Design review of the part built by this model. Coordinates are the model's own, in mm. Give positions to 0.01 mm unless a question says otherwise; leave off trailing zeros. Order: outer loops, then holes, each group sorted by start corner. A loop starts at its lowest first (then second) coordinate and runs counter-clockwise, first axis right, second up. Notation, with made-up numbers: (-3.75, 8) - (21.25, 8) arc R18 ccw to (21.25, 33) - close; hole circle Ø2 at (20.25, 53.25). An arc over 180 degrees is marked (long way). Write each question's results on one line, items separated by ' | '. Start each with the question number.
```python
from build123d import *

# Parameters (mm, degrees)
SKETCH1_W               = 510
SKETCH1_H               = 350
BOSS_EXTRUDE1_DEPTH     = 5
SKETCH2_R               = 5
SKETCH2_R_2             = 2.5
F_1_JOYYSTICK_DEPTH     = 619.566892098
SKETCH3_R               = 12
F_1_BUTTONS_DEPTH       = 619.566892098
SKETCH4_R               = 6.25
F_1_ROCKET_SWITCH_DEPTH = 619.566892098
SKETCH5_R               = 2.25
SKETCH5_W               = 2
SKETCH5_H               = 74
F_1_POTENTIOMETER_DEPTH = 619.566892098
FILLET1_R               = 35
SKETCH6_R               = 12
F_2_BUTTONS_DEPTH       = 619.566892098
SKETCH9_R               = 25
F_2_SPEAKER_DEPTH       = 619.566892098
SKETCH10_R              = 6.25
F_2_ROCKET_SWITCH_DEPTH = 619.566892098
SKETCH8_R               = 2
SKETCH8_W               = 2
SKETCH8_H               = 75
F_2_POTENTIOMETER_DEPTH = 619.566892098


with BuildPart() as part:
    # Sketch1 → Boss-Extrude1 (new body)
    with BuildSketch(Plane(origin=(0, 0, 0), x_dir=(1, 0, 0), z_dir=(0, 1, 0))):
        with Locations((255, 175)):
            Rectangle(SKETCH1_W, SKETCH1_H)
    extrude(amount=BOSS_EXTRUDE1_DEPTH)

    # Sketch2 → 1 Joyystick (cut, through all)
    with BuildSketch(Plane(origin=(0, 5, 0), x_dir=(1, 0, 0), z_dir=(0, 1, 0))):
        with Locations(Location((120, 250, 0), (0, 0, 270))):
            Circle(SKETCH2_R)
        with Locations(Location((162.5, 270, 0), (0, 0, 270))):
            Circle(SKETCH2_R_2)
        with Locations(Location((162.5, 230, 0), (0, 0, 90))):
            Circle(SKETCH2_R_2)
        with Locations(Location((77.5, 230, 0), (0, 0, 270))):
            Circle(SKETCH2_R_2)
        with Locations(Location((77.5, 270, 0), (0, 0, 90))):
            Circle(SKETCH2_R_2)
    extrude(amount=-F_1_JOYYSTICK_DEPTH, mode=Mode.SUBTRACT)

    # Sketch3 → 1 Buttons (cut, through all)
    with BuildSketch(Plane(origin=(0, 5, 0), x_dir=(1, 0, 0), z_dir=(0, 1, 0))):
        with Locations(Location((80, 180, 0), (0, 0, 270))):
            Circle(SKETCH3_R)
        with Locations(Location((130, 180, 0), (0, 0, 270))):
            Circle(SKETCH3_R)
        with Locations(Location((100, 130, 0), (0, 0, 270))):
            Circle(SKETCH3_R)
        with Locations(Location((150, 130, 0), (0, 0, 270))):
            Circle(SKETCH3_R)
        with Locations(Location((150, 80, 0), (0, 0, 270))):
            Circle(SKETCH3_R)
    extrude(amount=-F_1_BUTTONS_DEPTH, mode=Mode.SUBTRACT)

    # Sketch4 → 1 Rocket Switch (cut, through all)
    with BuildSketch(Plane(origin=(0, 5, 0), x_dir=(1, 0, 0), z_dir=(0, 1, 0))):
        with Locations(Location((190, 280, 0), (0, 0, 270))):
            Circle(SKETCH4_R)
    extrude(amount=-F_1_ROCKET_SWITCH_DEPTH, mode=Mode.SUBTRACT)

    # Sketch5 → 1 Potentiometer (cut, through all)
    with BuildSketch(Plane(origin=(0, 5, 0), x_dir=(1, 0, 0), z_dir=(0, 1, 0))):
        with Locations(Location((178.719749064, 192, 0), (0, 0, 270))):
            Circle(SKETCH5_R)
        with Locations(Location((192.718338039, 191.801237073, 0), (0, 0, 90))):
            Circle(SKETCH5_R)
        with Locations(Location((192.718338039, 108.198762927, 0), (0, 0, 270))):
            Circle(SKETCH5_R)
        with Locations(Location((178.719749064, 108, 0), (0, 0, 90))):
            Circle(SKETCH5_R)
        with Locations((191, 150)):
            Rectangle(SKETCH5_W, SKETCH5_H)
    extrude(amount=-F_1_POTENTIOMETER_DEPTH, mode=Mode.SUBTRACT)

    # Fillet1
    fillet1_edges = [part.edges().sort_by_distance(p)[0] for p in [
        (0, 2.5, -350),
        (510, 2.5, -350),
        (510, 2.5, 0),
        (0, 2.5, 0),
    ]]
    fillet(fillet1_edges, radius=FILLET1_R)

    # Sketch6 → 2 Buttons (cut, through all)
    with BuildSketch(Plane(origin=(0, 5, 0), x_dir=(1, 0, 0), z_dir=(0, 1, 0))):
        with Locations(Location((460, 200, 0), (0, 0, 270))):
            Circle(SKETCH6_R)
        with Locations(Location((410, 200, 0), (0, 0, 270))):
            Circle(SKETCH6_R)
        with Locations(Location((424.025675508, 150, 0), (0, 0, 270))):
            Circle(SKETCH6_R)
        with Locations(Location((374.025675508, 150, 0), (0, 0, 270))):
            Circle(SKETCH6_R)
        with Locations(Location((460, 110, 0), (0, 0, 270))):
            Circle(SKETCH6_R)
    extrude(amount=-F_2_BUTTONS_DEPTH, mode=Mode.SUBTRACT)

    # Sketch9 → 2 speaker (cut, through all)
    with BuildSketch(Plane(origin=(0, 5, 0), x_dir=(1, 0, 0), z_dir=(0, 1, 0))):
        with Locations(Location((410, 290, 0), (0, 0, 270))):
            Circle(SKETCH9_R)
    extrude(amount=-F_2_SPEAKER_DEPTH, mode=Mode.SUBTRACT)

    # Sketch10 → 2 Rocket Switch (cut, through all)
    with BuildSketch(Plane(origin=(0, 5, 0), x_dir=(1, 0, 0), z_dir=(0, 1, 0))):
        with Locations(Location((370, 80, 0), (0, 0, 270))):
            Circle(SKETCH10_R)
    extrude(amount=-F_2_ROCKET_SWITCH_DEPTH, mode=Mode.SUBTRACT)

    # Sketch8 → 2 Potentiometer (cut, through all)
    with BuildSketch(Plane(origin=(0, 5, 0), x_dir=(1, 0, 0), z_dir=(0, 1, 0))):
        with Locations(Location((320, 192.5, 0), (0, 0, 270))):
            Circle(SKETCH8_R)
        with Locations(Location((320, 107.5, 0), (0, 0, 90))):
            Circle(SKETCH8_R)
        with Locations(Location((306, 107.5, 0), (0, 0, 270))):
            Circle(SKETCH8_R)
        with Locations(Location((306, 192.5, 0), (0, 0, 90))):
            Circle(SKETCH8_R)
        with Locations((308, 150)):
            Rectangle(SKETCH8_W, SKETCH8_H)
    extrude(amount=-F_2_POTENTIOMETER_DEPTH, mode=Mode.SUBTRACT)


solid = part.part
```
Q1. For line 1 (X direction, y = 2.1, z = -151); line 2 (Z direction, x = 162.5, y = 3.8); line 3 (X direction, y = 2.5, z = -230), list the stretches that pass through material, from the lowest coordinate up. Write a range as [from, to].
Q2. Add section A-A (x = 150). Give the boundary of the cut face in (y, z).
Q3. Add section B-B (z = -130). Give the boundary of the cut face in (x, y).
Q4. Add section C-C (z = -200). Give the boundary of the cut face in (x, y), plus the area to 3 significant figures.
Q5. Draft analysis for pull direction Z (two halves, no side actions). For faces 1 (the cylindrical face through (499.475, 2.535, -9.981)), 2 (the flat face through (251, 0, -177)), 3 (the cylindrical face through (468.11, 2.535, -118.844)), 4 (the cylindrical face through (499.475, 2.535, -340.019)), state which applies: pulls with the +Z half, pulls with the -Z half, needs draft (parallel to the pull), parting line crosses it, or undercut.
Q6. Insertion check: pin 1 Ø2.5 at (x, z) = (178.72, -108) entering from -Y. The pin has a flat end and moves straight along its axis. Give the tip position at first contact, or say it passes through.
Q7. Add section D-D (z = -296). Give the boundary of the cut face in (x, y).
Verdict:
1) line 1: x = [0, 190], [192, 307], [309, 362.07], [385.98, 412.07], [435.98, 510] | line 2: z = [-350, -272.5], [-267.5, -232.5], [-227.5, 0] | line 3: x = [0, 75], [80, 160], [165, 510]
2) outline: (0, -350) - (5, -350) - (5, -142) - (0, -142) - close; (0, -118) - (5, -118) - (5, -92) - (0, -92) - close; (0, -68) - (5, -68) - (5, 0) - (0, 0) - close
3) outline: (0, 0) - (88, 0) - (88, 5) - (0, 5) - close; (112, 0) - (138, 0) - (138, 5) - (112, 5) - close; (162, 0) - (190, 0) - (190, 5) - (162, 5) - close; (192, 0) - (307, 0) - (307, 5) - (192, 5) - close; (309, 0) - (510, 0) - (510, 5) - (309, 5) - close
4) outline: (0, 0) - (398, 0) - (398, 5) - (0, 5) - close; (422, 0) - (448, 0) - (448, 5) - (422, 5) - close; (472, 0) - (510, 0) - (510, 5) - (472, 5) - close | area: 2,310 mm2
5) face 1: pulls with the +Z half | face 2: needs draft | face 3: undercut | face 4: pulls with the -Z half
6) pin 1: passes through
7) outline: (0, 0) - (385.73, 0) - (385.73, 5) - (0, 5) - close; (434.27, 0) - (510, 0) - (510, 5) - (434.27, 5) - close
